Autodesk Inventor part; units mm, degrees
ref_plane "YZ Plane" through (0, 0, 0) normal (1, 0, 0) x (0, 1, 0)
ref_plane "XZ Plane" through (0, 0, 0) normal (0, 1, 0) x (-1, 0, 0)
ref_plane "XY Plane" through (0, 0, 0) normal (0, 0, 1) x (1, 0, 0)
sketch "Эскиз1" plane through (0, 0, 0) normal (0, 0, 1) x (1, 0, 0)
  line L0 (0, 0) -> (118.4333, 0)
  line L1 (0, 28.5) -> (4, 28.5)
  line L2 (4, 28.5) -> (4, 36)
  line L3 (0, 28.5) -> (0, 50)
  line L4 (0, 50) -> (9, 50)
  line L5 (9, 50) -> (9, 54)
  line L6 (9, 54) -> (15, 54)
  line L7 (15, 54) -> (15, 47.5)
  line L8 (4, 36) -> (12, 36)
  line L9 (15, 47.5) -> (18, 47.5)
  line L10 (18, 47.5) -> (18, 44.5)
  line L11 (18, 44.5) -> (14.1429, 44.5)
  line L12 (14.1429, 44.5) -> (14.1429, 36)
  line L13 (14.1429, 36) -> (12, 36)
  dimension "d0" = 57
  dimension "d1" = 100
  dimension "d3" = 6
  dimension "d4" = 4
  dimension "d6" = 72
  dimension "d7" = 8
  dimension "d8" = 4
  dimension "d10" = 3
  dimension "d11" = 95
  dimension "d13" = 9
  dimension "d17" = 3
revolve "Вращение1" add sketch "Эскиз1" angle 360 about axis through (0, 0, 0) along (1, 0, 0)
chamfer "Фаска1" distance 1 angle 45 1 edges at (0, -50, 0)
properties part number "Крышка_Левая" material "Сталь, углеродистая"
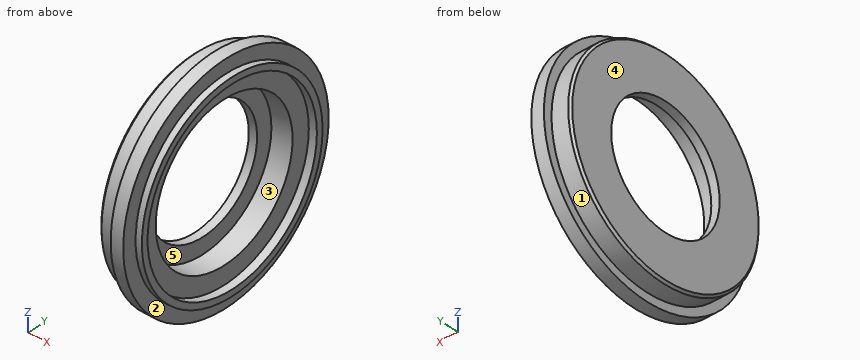
For this review, take the finished solid that the model builds, in its own axes (mm). Face numbers are marked on the shaded views. A direction names the side the tool comes from. Round coordinates to 2 decimals unless told otherwise and drop trailing zeros. Write each loop counter-clockwise with the first axis right and the second up, starting at its lowest first coordinate (ties: lowest second). Pieces come first, ordered by that corner, then holes. Notation, with made-up numbers: (58.5, 4.5) - (78.5, 4.5) arc R32 cw to (78.5, 33.5) - close; hole circle Ø7 at (20, -37.75). An arc over 180 degrees is marked (long way). Answer as a JSON object with one key per item and string values.
1. Draft analysis for pull direction Y (two halves, no side actions). For the marked faces 1, 2 and 3, state which applies: +Y half, -Y half, draft (parallel to the pull), parting line (faces both ways), or undercut.
Response values:
{"face 1": "parting line", "face 2": "draft", "face 3": "undercut"}
2. We need section A-A on y = 0. Give the boundary of the cut face in (x, z).
Response values:
{"outline": "(0, -49) - (1, -50) - (9, -50) - (9, -54) - (15, -54) - (15, -47.5) - (18, -47.5) - (18, -44.5) - (14.14, -44.5) - (14.14, -36) - (4, -36) - (4, -28.5) - (0, -28.5) - close; (0, 28.5) - (4, 28.5) - (4, 36) - (14.14, 36) - (14.14, 44.5) - (18, 44.5) - (18, 47.5) - (15, 47.5) - (15, 54) - (9, 54) - (9, 50) - (1, 50) - (0, 49) - close"}
3. We need section C-C on x = 11. Give the boundary of the cut face in (y, z), then the cut area to 3 significant figures.
Response values:
{"outline": "circle Ø108 at (0, 0); hole circle Ø72 at (0, 0)", "area": "5,090 mm2"}
4. To check wall thickness, follow line 1 along Z through (x, y) = (12, 0); line 2 along Z through (x, y) = (16.3, 0); line 3 along X through (y, z) = (9, 29.5). State the ranges of each line that lie inside material, in increasing order.
Response values:
{"line 1": "z = -54 to -36, 36 to 54", "line 2": "z = -47.5 to -44.5, 44.5 to 47.5", "line 3": "x = 0 to 4"}
5. Tool access review of the marked faces 4 and 5: name each direction out of +Z, -Z, +X, -X, +Y, -Y from which nothing blocks a thin tool from reaching the whole face with its end or side.
Response values:
{"face 4": "+Z, -Z, -X, +Y, -Y", "face 5": "+X"}
6. For pin 1 Ø1.5 at (x, y) = (2, -31) entering from +Z; pin 2 Ø2 at (x, y) = (12, -10.5) entering from -Z; pin 3 Ø3 at (x, y) = (3.5, 18.5) entering from -Z, all flat-tipped, find the tip position at first contact; note any pin that passes through.
Response values:
{"pin 1": "stops at z = 39.81", "pin 2": "stops at z = -53.16", "pin 3": "stops at z = -47.02"}
